The drawing under review shows one solid part. Ordinate dimensions are in mm from its lowest x, y, z. A direction names the side the tool comes from. Give positions to 0.01 mm unless a question says otherwise; leave off trailing zeros. Write each loop counter-clockwise with the first axis right and the second up, starting at its lowest first coordinate (ties: lowest second). Pieces come first, ordered by that corner, then holes. Notation, with made-up numbers: M 14.5,-31 L 60.5,-31 A15 ccw 60.5,-13 Z; hole C 82.25,8 d4. An arc over 180 degrees is marked long. Write item = value, one per line. Start each with the question number.
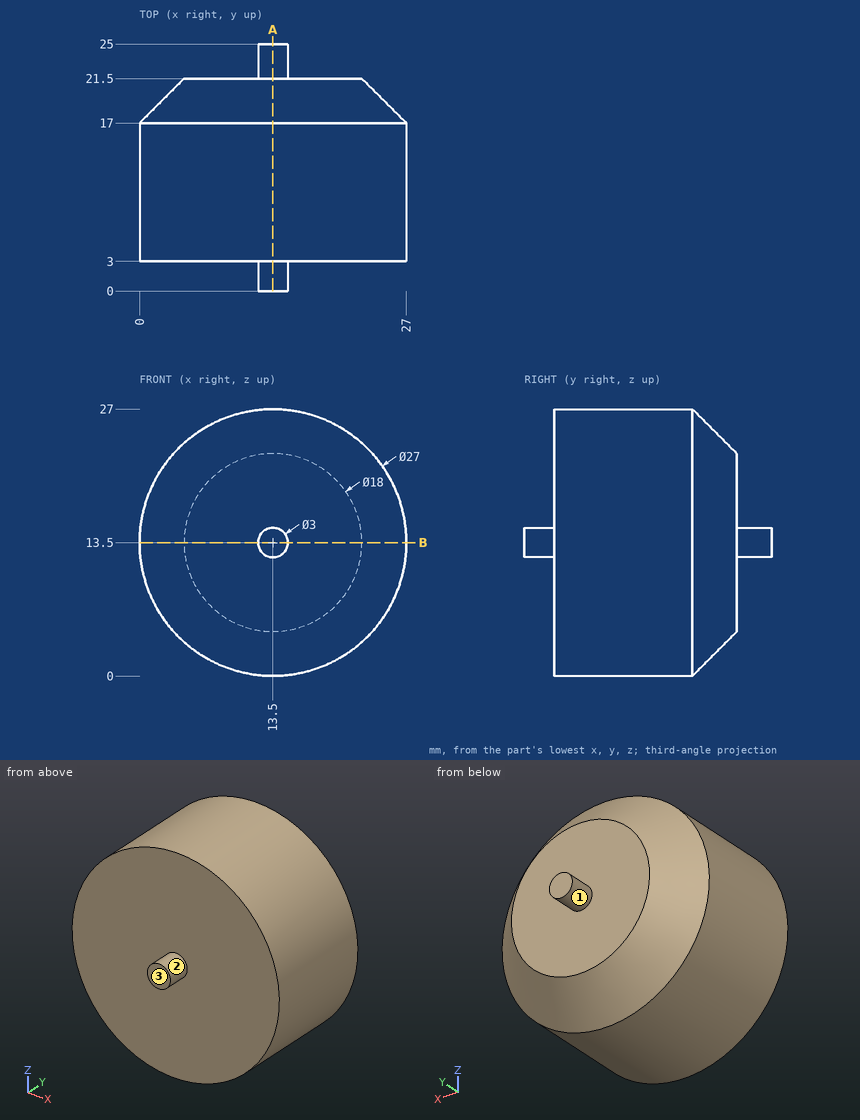
Item 1: Clearance check with flat-ended pins moving along their axes: P1, Ø4, axis at x = 19.5, z = 9, coming from the +Y side; P2, Ø1, axis at x = 7, y = 12.5, coming from the -Z side; P3, Ø8, axis at x = 10, z = 10, coming from the -Y side; P4, Ø1.5, axis at x = 24, y = 8, coming from the -Z side. State where each tip first meets the part, or that it passes through.
Item 2: We need section A-A, the plane x = 13.5. Write out the cut boundary in (y, z).
Item 3: We need section B-B, the plane z = 13.5. Write out the cut boundary in (x, y).
Item 4: For the marked faces 1, 2 and 3, list the 3-axis set-ups (+Z, -Z, +X, -X, +Y, -Y) from which the entire face can be reached by the end or side of a thin tool; tool diameter is ignored.
Item 5: To check wall thickness, follow probe 1 along Y at (x, z) = (15, 11.75); probe 2 along Z at (x, y) = (14.5, 17); probe 3 along X at (y, z) = (19.25, 20.25). State the ranges of each line that lie inside material, in increasing order. Write a range as [from, to].
Worked out:
q1.P1 = 21.5
q1.P2 = 1.41
q1.P3 = 0
q1.P4 = 4.16
q2.outline = M 0,12 L 3,12 L 3,0 L 17,0 L 21.5,4.5 L 21.5,12 L 25,12 L 25,15 L 21.5,15 L 21.5,22.5 L 17,27 L 3,27 L 3,15 L 0,15 Z
q3.outline = M 0,3 L 12,3 L 12,0 L 15,0 L 15,3 L 27,3 L 27,17 L 22.5,21.5 L 15,21.5 L 15,25 L 12,25 L 12,21.5 L 4.5,21.5 L 0,17 Z
q4.face_1 = +Y
q4.face_2 = -Y
q4.face_3 = +Z, -Z, +X, -X, -Y
q5.probe_1 = [3, 21.5]
q5.probe_2 = [0.04, 26.96]
q5.probe_3 = [4.5, 22.5]
